For this review, take the finished solid that the model builds, in its own axes (mm). Face numbers are marked on the shaded views. A direction names the side the tool comes from. Round coordinates to 2 decimals unless told otherwise and drop trailing zeros. Write each loop counter-clockwise with the first axis right and the second up, starting at its lowest first coordinate (ties: lowest second). Pieces come first, ordered by that corner, then holes. Notation, with made-up numbers: M 86,-2 L 144,-2 A27 cw 144,25 Z; hole C 17.5,-1.5 d11. An arc over 180 degrees is marked long. Use one line per item in the form item = value. Start each with the question number.
Item 1: For line 1 (Z direction, x = 2.25, y = -0.25); line 2 (Z direction, x = 1, y = -1); line 3 (Y direction, x = 0.5, z = 1.5), list the stretches that pass through material, from the lowest coordinate up. Write a range as [from, to].
Item 2: For P1, Ø0.9, axis at x = -0.5, y = 0.5, coming from the +Z side; P2, Ø2, axis at y = -1.5, z = 6.5, coming from the +X side; P3, Ø2, axis at x = 1.5, y = 1, coming from the -Z side; P4, Ø1, axis at x = -1.5, z = 17, coming from the -Y side, all flat-tipped, find the tip position at first contact; note any pin that passes through.
Item 3: Draft analysis for pull direction X (two halves, no side actions). For the marked faces 3, 4 and 5, state which applies: released by +X, released by -X, zero draft, split by the parting line, or undercut.
Item 4: Add section A-A (z = 19.5). State the section outline as (x, y) points, and give its area (3 significant figures).
Item 5: For the marked faces 1 and 2, list the 3-axis set-ups (+Z, -Z, +X, -X, +Y, -Y) from which the entire face can be reached by the end or side of a thin tool; tool diameter is ignored.
Autodesk Inventor part; units mm, degrees
ref_plane "YZ Plane" through (0, 0, 0) normal (1, 0, 0) x (0, 1, 0)
ref_plane "XZ Plane" through (0, 0, 0) normal (0, 1, 0) x (-1, 0, 0)
ref_plane "XY Plane" through (0, 0, 0) normal (0, 0, 1) x (1, 0, 0)
sketch "Sketch1" plane through (0, 0, 0) normal (0, 0, 1) x (1, 0, 0)
  circle A0 centre (0, 0) radius 2
  dimension "Diameter" = 4
extrude "Extrusion1" add sketch "Sketch1" along normal blind 20
sketch "Sketch2" plane through (0, 0, 20) normal (0, 0, 1) x (1, 0, 0)
  circle A0 centre (0, 0) radius 2
  circle A1 centre (0, 0) radius 3.5
  dimension "Head_Diameter" = 7
extrude "Extrusion2" add sketch "Sketch2" along normal blind 4 contours A0 | A1
sketch "Sketch3" plane through (0, 0, 24) normal (0, 0, 1) x (1, 0, 0)
  circle A0 centre (0, 0) radius 3.5
  circle A1 centre (0, 0) radius 1.7321 construction
  line L0 (0, 1.7321) -> (1.5, 0.866)
  line L1 (1.5, -0.866) -> (1.5, 0.866)
  line L2 (0, 1.7321) -> (-1.5, 0.866)
  line L3 (-1.5, -0.866) -> (-1.5, 0.866)
  line L4 (-1.5, -0.866) -> (0, -1.7321)
  line L5 (1.5, -0.866) -> (0, -1.7321)
  dimension "Hex_Width" = 3
extrude "Extrusion3" cut sketch "Sketch3" against normal blind 2 contours L0 L1 L5 L4 L3 L2
thread "Thread1"
chamfer "Chamfer1" distance 0.4 angle 45 2 edges at (-3.5, 0, 24) (-2, 0, 0)
equation "\"d9\" = ThreadLength"
equation "\"d12\" = Chamfer"
equation "\"ThreadLength\" = 20"
properties part number "SCREW, SOCKET HD, P, 12_9, M4X0_7X20" material "Steel, MS"
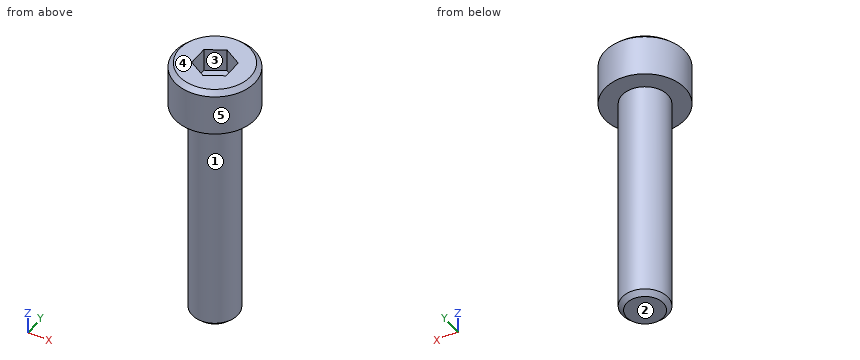
Calculated:
q1.line_1 = [20, 24]
q1.line_2 = [0, 22]
q1.line_3 = [-1.94, 1.94]
q2.P1 = 22
q2.P2 = 1.94
q2.P3 = 0
q2.P4 = -1.73
q3.face_3 = undercut
q3.face_4 = zero draft
q3.face_5 = split by the parting line
q4.outline = C 0,0 d4
q4.area = 12.6 mm^2
q5.face_1 = -Z
q5.face_2 = -Z, +X, -X, +Y, -Y
